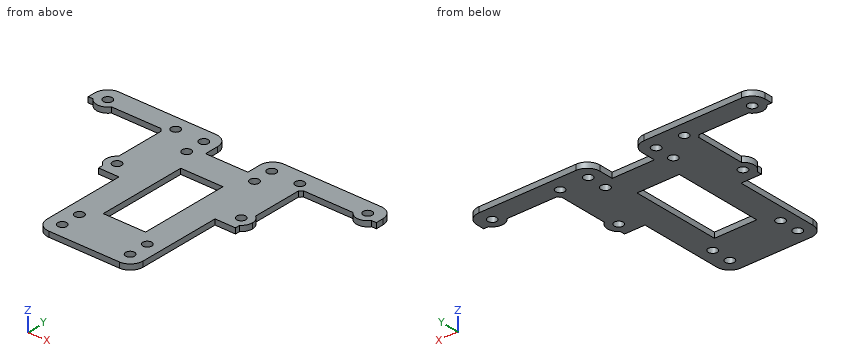
from build123d import *

# Parameters (mm, degrees)
F0_R     = 1.778
F0_W     = 16.764
F0_H     = 35.56
F1_DEPTH = 2.159
F2_R     = 5.08


with BuildPart() as f1:
    # F0 (on Top) → F1 (new body)
    with BuildSketch(Plane.XY):
        with BuildLine():
            Line((57.15, 10.922), (57.15, 19.05))
            Line((57.15, 19.05), (8.382, 19.05))
            Line((8.382, 19.05), (8.382, 8.382))
            Line((8.382, 8.382), (-8.382, 8.382))
            Line((-8.382, 8.382), (-8.382, 19.05))
            Line((-8.382, 19.05), (-57.15, 19.05))
            Line((-57.15, 19.05), (-57.15, 10.922))
            Line((-57.15, 10.922), (-55.209797, 10.922))
            ThreePointArc((-55.209797, 10.922), (-52.893083, 17.703019), (-47.117, 13.462))
            ThreePointArc((-47.117, 13.462), (-47.320981, 12.130917), (-47.914203, 10.922))
            Line((-47.914203, 10.922), (-28.285797, 10.922))
            ThreePointArc((-28.285797, 10.922), (-25.969083, 17.703019), (-20.193, 13.462))
            ThreePointArc((-20.193, 13.462), (-22.580365, 9.521929), (-27.178, 9.814203))
            Line((-27.178, 9.814203), (-27.178, -9.814203))
            ThreePointArc((-27.178, -9.814203), (-22.580365, -9.521929), (-20.193, -13.462))
            ThreePointArc((-20.193, -13.462), (-22.580365, -17.402071), (-27.178, -17.109797))
            Line((-27.178, -17.109797), (-27.178, -19.05))
            Line((-27.178, -19.05), (-19.05, -19.05))
            Line((-19.05, -19.05), (-19.05, -57.15))
            Line((-19.05, -57.15), (19.05, -57.15))
            Line((19.05, -57.15), (19.05, -19.05))
            Line((19.05, -19.05), (27.178, -19.05))
            Line((27.178, -19.05), (27.178, -17.109797))
            ThreePointArc((27.178, -17.109797), (20.193, -13.462), (27.178, -9.814203))
            Line((27.178, -9.814203), (27.178, 9.814203))
            ThreePointArc((27.178, 9.814203), (20.697929, 15.519635), (29.083, 13.462))
            ThreePointArc((29.083, 13.462), (28.879019, 12.130917), (28.285797, 10.922))
            Line((28.285797, 10.922), (47.914203, 10.922))
            ThreePointArc((47.914203, 10.922), (50.230917, 17.703019), (56.007, 13.462))
            ThreePointArc((56.007, 13.462), (55.803019, 12.130917), (55.209797, 10.922))
            Line((55.209797, 10.922), (57.15, 10.922))
        make_face()
        with Locations((-13.462, -51.562)):
            Circle(F0_R, mode=Mode.SUBTRACT)
        with Locations((-13.462, -43.688)):
            Circle(F0_R, mode=Mode.SUBTRACT)
        with Locations((13.462, -51.562)):
            Circle(F0_R, mode=Mode.SUBTRACT)
        with Locations((13.462, -43.688)):
            Circle(F0_R, mode=Mode.SUBTRACT)
        with Locations((0, -20.828)):
            Rectangle(F0_W, F0_H, mode=Mode.SUBTRACT)
        with Locations((-13.462, 5.588)):
            Circle(F0_R, mode=Mode.SUBTRACT)
        with Locations((-13.462, 13.462)):
            Circle(F0_R, mode=Mode.SUBTRACT)
        with Locations((13.462, 5.588)):
            Circle(F0_R, mode=Mode.SUBTRACT)
        with Locations((13.462, 13.462)):
            Circle(F0_R, mode=Mode.SUBTRACT)
        with BuildLine():
            ThreePointArc((47.914203, 10.922), (51.562, 9.017), (55.209797, 10.922))
            ThreePointArc((55.209797, 10.922), (55.803019, 12.130917), (56.007, 13.462))
            ThreePointArc((56.007, 13.462), (50.230917, 17.703019), (47.914203, 10.922))
        make_face()
        with Locations((51.562, 13.462)):
            Circle(F0_R, mode=Mode.SUBTRACT)
        with BuildLine():
            ThreePointArc((27.178, 9.814203), (27.78109, 10.31891), (28.285797, 10.922))
            ThreePointArc((28.285797, 10.922), (28.879019, 12.130917), (29.083, 13.462))
            ThreePointArc((29.083, 13.462), (20.697929, 15.519635), (27.178, 9.814203))
        make_face()
        with Locations((24.638, 13.462)):
            Circle(F0_R, mode=Mode.SUBTRACT)
        with BuildLine():
            ThreePointArc((29.083, -13.462), (28.578071, -11.404365), (27.178, -9.814203))
            ThreePointArc((27.178, -9.814203), (20.193, -13.462), (27.178, -17.109797))
            ThreePointArc((27.178, -17.109797), (28.578071, -15.519635), (29.083, -13.462))
        make_face()
        with Locations((24.638, -13.462)):
            Circle(F0_R, mode=Mode.SUBTRACT)
        with BuildLine():
            ThreePointArc((-47.117, 13.462), (-52.893083, 17.703019), (-55.209797, 10.922))
            ThreePointArc((-55.209797, 10.922), (-51.562, 9.017), (-47.914203, 10.922))
            ThreePointArc((-47.914203, 10.922), (-47.320981, 12.130917), (-47.117, 13.462))
        make_face()
        with Locations((-51.562, 13.462)):
            Circle(F0_R, mode=Mode.SUBTRACT)
        with BuildLine():
            ThreePointArc((-20.193, 13.462), (-25.969083, 17.703019), (-28.285797, 10.922))
            ThreePointArc((-28.285797, 10.922), (-27.78109, 10.31891), (-27.178, 9.814203))
            ThreePointArc((-27.178, 9.814203), (-22.580365, 9.521929), (-20.193, 13.462))
        make_face()
        with Locations((-24.638, 13.462)):
            Circle(F0_R, mode=Mode.SUBTRACT)
        with BuildLine():
            ThreePointArc((-20.193, -13.462), (-22.580365, -9.521929), (-27.178, -9.814203))
            ThreePointArc((-27.178, -9.814203), (-29.083, -13.462), (-27.178, -17.109797))
            ThreePointArc((-27.178, -17.109797), (-22.580365, -17.402071), (-20.193, -13.462))
        make_face()
        with Locations((-24.638, -13.462)):
            Circle(F0_R, mode=Mode.SUBTRACT)
    extrude(amount=F1_DEPTH)

    # F2
    f2_edges = [f1.edges().sort_by_distance(p)[0] for p in [
        (57.15, 19.05, 1.0795),
        (8.382, 19.05, 1.0795),
        (-8.382, 19.05, 1.0795),
        (19.05, -57.15, 1.0795),
        (-19.05, -57.15, 1.0795),
        (-57.15, 19.05, 1.0795),
    ]]
    fillet(f2_edges, radius=F2_R)


solid = f1.part
Can you work these out from the model? Positions are in its coordinate system, mm. Coordinates: 2 decimals unless noted, no trailing zeros. Write each loop counter-clockwise with the first axis right and the second up, starting at its lowest first coordinate (ties: lowest second). Pieces come first, ordered by that corner, then holes.
Q1. For P1, Ø0.6, axis at y = -33.5, z = 1, coming from the +X side; P2, Ø3, axis at x = -13.462, y = 5.588, coming from the +Z side; P3, Ø0.6, axis at y = -28.5, z = 0.5, coming from the -X side, each with a flat end and sliding along its axis, tell me the tip position at first contact or that it passes through.
Results found:
P1: stops at x = 19.05
P2: passes through
P3: stops at x = -19.05
Q2. Imagine slicing it at D-D, the plane z = 1.7. Count the separate pieces of the cut face and the enclosed holes in it, plus the area to 3 significant figures.
Results found:
separate pieces: 1
enclosed holes: 15
area: 3,100 mm2
Q3. Imagine slicing it at C-C, the plane y = -47. List the corners of the cut face in (x, z) for me, plus the area to 3 significant figures.
Results found:
outline: (-19.05, 0) - (19.05, 0) - (19.05, 2.16) - (-19.05, 2.16) - close
area: 82.3 mm2
Q4. Please list where these lines run through material, in increasing order: L1, parallel to X at y = -51.5, z = 0.4; L2, parallel to X at y = -5, z = 1.05; L3, parallel to Y at x = -5, z = 1.4.
Results found:
L1: x = -19.05 to -15.24, -11.69 to 11.69, 15.24 to 19.05
L2: x = -27.18 to -8.38, 8.38 to 27.18
L3: y = -57.15 to -38.61, -3.05 to 8.38
Q5. Imagine slicing it at B-B, the plane x = 5. List the corners of the cut face in (y, z) for me, plus the area to 3 significant figures.
Results found:
outline: (-57.15, 0) - (-38.61, 0) - (-38.61, 2.16) - (-57.15, 2.16) - close; (-3.05, 0) - (8.38, 0) - (8.38, 2.16) - (-3.05, 2.16) - close
area: 64.7 mm2
Q6. Imagine slicing it at A-A, the plane y = -5. List the corners of the cut face in (x, z) for me.
Results found:
outline: (-27.18, 0) - (-8.38, 0) - (-8.38, 2.16) - (-27.18, 2.16) - close; (8.38, 0) - (27.18, 0) - (27.18, 2.16) - (8.38, 2.16) - close
